from build123d import *

# Parameters (mm, degrees)
F0_R      = 3
F0_R_2    = 15
F1_DEPTH  = 12
F2_R      = 6
F3_DEPTH  = 6
F4_R      = 2
F5_DEPTH  = 12.001
F6_R      = 35
F7_DEPTH  = 4
F8_R      = 35
F9_DEPTH  = 4
F10_R     = 2
F11_DEPTH = 25


with BuildPart() as f1:
    # F0 (on Top) → F1 (new body)
    with BuildSketch(Plane.XY):
        with BuildLine():
            Line((7, 55.425626), (7, 100))
            ThreePointArc((7, 100), (0, 107), (-7, 100))
            Line((-7, 100), (-7, 55.425626))
            ThreePointArc((-7, 55.425626), (-19.5, 33.774991), (-44.5, 33.774991))
            Line((-44.5, 33.774991), (-83.10254, 56.062178))
            ThreePointArc((-83.10254, 56.062178), (-92.664718, 53.5), (-90.10254, 43.937822))
            Line((-90.10254, 43.937822), (-51.5, 21.650635))
            ThreePointArc((-51.5, 21.650635), (-39, 0), (-51.5, -21.650635))
            Line((-51.5, -21.650635), (-90.10254, -43.937822))
            ThreePointArc((-90.10254, -43.937822), (-92.664718, -53.5), (-83.10254, -56.062178))
            Line((-83.10254, -56.062178), (-44.5, -33.774991))
            ThreePointArc((-44.5, -33.774991), (-19.5, -33.774991), (-7, -55.425626))
            Line((-7, -55.425626), (-7, -100))
            ThreePointArc((-7, -100), (0, -107), (7, -100))
            Line((7, -100), (7, -55.425626))
            ThreePointArc((7, -55.425626), (19.5, -33.774991), (44.5, -33.774991))
            Line((44.5, -33.774991), (83.10254, -56.062178))
            ThreePointArc((83.10254, -56.062178), (92.664718, -53.5), (90.10254, -43.937822))
            Line((90.10254, -43.937822), (51.5, -21.650635))
            ThreePointArc((51.5, -21.650635), (39, 0), (51.5, 21.650635))
            Line((51.5, 21.650635), (90.10254, 43.937822))
            ThreePointArc((90.10254, 43.937822), (92.664718, 53.5), (83.10254, 56.062178))
            Line((83.10254, 56.062178), (44.5, 33.774991))
            ThreePointArc((44.5, 33.774991), (19.5, 33.774991), (7, 55.425626))
        make_face()
        with Locations((-86.60254, -50)):
            Circle(F0_R, mode=Mode.SUBTRACT)
        with Locations((-38.971143, -22.5)):
            Circle(F0_R, mode=Mode.SUBTRACT)
        with Locations((0, -100)):
            Circle(F0_R, mode=Mode.SUBTRACT)
        with Locations((0, -45)):
            Circle(F0_R, mode=Mode.SUBTRACT)
        Circle(F0_R_2, mode=Mode.SUBTRACT)
        with Locations((38.971143, -22.5)):
            Circle(F0_R, mode=Mode.SUBTRACT)
        with Locations((86.60254, -50)):
            Circle(F0_R, mode=Mode.SUBTRACT)
        with Locations((-86.60254, 50)):
            Circle(F0_R, mode=Mode.SUBTRACT)
        with Locations((-38.971143, 22.5)):
            Circle(F0_R, mode=Mode.SUBTRACT)
        with Locations((38.971143, 22.5)):
            Circle(F0_R, mode=Mode.SUBTRACT)
        with Locations((0, 45)):
            Circle(F0_R, mode=Mode.SUBTRACT)
        with Locations((86.60254, 50)):
            Circle(F0_R, mode=Mode.SUBTRACT)
        with Locations((0, 100)):
            Circle(F0_R, mode=Mode.SUBTRACT)
    extrude(amount=F1_DEPTH)

    # F2 (on face) → F3 (cut)
    with BuildSketch(Plane.XY.offset(12)):
        with Locations((-86.60254, 50)):
            Circle(F2_R)
        with Locations((0, 100)):
            Circle(F2_R)
        with Locations((86.60254, 50)):
            Circle(F2_R)
        with Locations((86.60254, -50)):
            Circle(F2_R)
        with Locations((0, -100)):
            Circle(F2_R)
        with Locations((-86.60254, -50)):
            Circle(F2_R)
        with Locations((-38.971143, 22.5)):
            Circle(F2_R)
        with Locations((0, 45)):
            Circle(F2_R)
        with Locations((38.971143, 22.5)):
            Circle(F2_R)
        with Locations((38.971143, -22.5)):
            Circle(F2_R)
        with Locations((0, -45)):
            Circle(F2_R)
        with Locations((-38.971143, -22.5)):
            Circle(F2_R)
    extrude(amount=-F3_DEPTH, mode=Mode.SUBTRACT)

    # F4 (on face) → F5 (cut, through all)
    with BuildSketch(Plane.XY.offset(12)):
        with Locations((0, 20)):
            Circle(F4_R)
        with Locations((-20, 0)):
            Circle(F4_R)
        with Locations((0, -20)):
            Circle(F4_R)
        with Locations((20, 0)):
            Circle(F4_R)
    extrude(amount=-F5_DEPTH, mode=Mode.SUBTRACT)

    # F6 (on face) → F7 (cut)
    with BuildSketch(Plane.XY.offset(12)):
        Circle(F6_R)
        with BuildLine():
            ThreePointArc((0, 93), (-3.535534, 91.535534), (-5, 88))
            Line((-5, 88), (-5, 57))
            ThreePointArc((-5, 57), (-3.535534, 53.464466), (0, 52))
            ThreePointArc((0, 52), (3.535534, 53.464466), (5, 57))
            Line((5, 57), (5, 88))
            ThreePointArc((5, 88), (3.535534, 91.535534), (0, 93))
        make_face()
        with BuildLine():
            Line((-46.863448, 32.830127), (-73.710236, 48.330127))
            ThreePointArc((-73.710236, 48.330127), (-77.504331, 48.829629), (-80.540363, 46.5))
            ThreePointArc((-80.540363, 46.5), (-81.039865, 42.705905), (-78.710236, 39.669873))
            Line((-78.710236, 39.669873), (-51.863448, 24.169873))
            ThreePointArc((-51.863448, 24.169873), (-48.069353, 23.670371), (-45.033321, 26))
            ThreePointArc((-45.033321, 26), (-44.533819, 29.794095), (-46.863448, 32.830127))
        make_face()
        with BuildLine():
            Line((-51.863448, -24.169873), (-78.710236, -39.669873))
            ThreePointArc((-78.710236, -39.669873), (-81.039865, -42.705905), (-80.540363, -46.5))
            ThreePointArc((-80.540363, -46.5), (-77.504331, -48.829629), (-73.710236, -48.330127))
            Line((-73.710236, -48.330127), (-46.863448, -32.830127))
            ThreePointArc((-46.863448, -32.830127), (-44.533819, -29.794095), (-45.033321, -26))
            ThreePointArc((-45.033321, -26), (-48.069353, -23.670371), (-51.863448, -24.169873))
        make_face()
        with BuildLine():
            Line((-5, -57), (-5, -88))
            ThreePointArc((-5, -88), (-3.535534, -91.535534), (0, -93))
            ThreePointArc((0, -93), (3.535534, -91.535534), (5, -88))
            Line((5, -88), (5, -57))
            ThreePointArc((5, -57), (3.535534, -53.464466), (0, -52))
            ThreePointArc((0, -52), (-3.535534, -53.464466), (-5, -57))
        make_face()
        with BuildLine():
            Line((46.863448, -32.830127), (73.710236, -48.330127))
            ThreePointArc((73.710236, -48.330127), (77.504331, -48.829629), (80.540363, -46.5))
            ThreePointArc((80.540363, -46.5), (81.039865, -42.705905), (78.710236, -39.669873))
            Line((78.710236, -39.669873), (51.863448, -24.169873))
            ThreePointArc((51.863448, -24.169873), (48.069353, -23.670371), (45.033321, -26))
            ThreePointArc((45.033321, -26), (44.533819, -29.794095), (46.863448, -32.830127))
        make_face()
        with BuildLine():
            Line((51.863448, 24.169873), (78.710236, 39.669873))
            ThreePointArc((78.710236, 39.669873), (81.039865, 42.705905), (80.540363, 46.5))
            ThreePointArc((80.540363, 46.5), (77.504331, 48.829629), (73.710236, 48.330127))
            Line((73.710236, 48.330127), (46.863448, 32.830127))
            ThreePointArc((46.863448, 32.830127), (44.533819, 29.794095), (45.033321, 26))
            ThreePointArc((45.033321, 26), (48.069353, 23.670371), (51.863448, 24.169873))
        make_face()
    extrude(amount=-F7_DEPTH, mode=Mode.SUBTRACT)

    # F8 (on face) → F9 (cut)
    with BuildSketch(Plane(origin=(0, 0, 0), x_dir=(1, 0, 0), z_dir=(0, 0, -1))):
        Circle(F8_R)
        with BuildLine():
            ThreePointArc((-73.710236, 48.330127), (-80.540363, 46.5), (-78.710236, 39.669873))
            Line((-78.710236, 39.669873), (-51.863448, 24.169873))
            ThreePointArc((-51.863448, 24.169873), (-45.033321, 26), (-46.863448, 32.830127))
            Line((-46.863448, 32.830127), (-73.710236, 48.330127))
        make_face()
        with BuildLine():
            ThreePointArc((-78.710236, -39.669873), (-80.540363, -46.5), (-73.710236, -48.330127))
            Line((-73.710236, -48.330127), (-46.863448, -32.830127))
            ThreePointArc((-46.863448, -32.830127), (-45.033321, -26), (-51.863448, -24.169873))
            Line((-51.863448, -24.169873), (-78.710236, -39.669873))
        make_face()
        with BuildLine():
            ThreePointArc((5, -57), (0, -52), (-5, -57))
            Line((-5, -57), (-5, -88))
            ThreePointArc((-5, -88), (0, -93), (5, -88))
            Line((5, -88), (5, -57))
        make_face()
        with BuildLine():
            ThreePointArc((73.710236, -48.330127), (80.540363, -46.5), (78.710236, -39.669873))
            Line((78.710236, -39.669873), (51.863448, -24.169873))
            ThreePointArc((51.863448, -24.169873), (45.033321, -26), (46.863448, -32.830127))
            Line((46.863448, -32.830127), (73.710236, -48.330127))
        make_face()
        with BuildLine():
            ThreePointArc((78.710236, 39.669873), (80.540363, 46.5), (73.710236, 48.330127))
            Line((73.710236, 48.330127), (46.863448, 32.830127))
            ThreePointArc((46.863448, 32.830127), (45.033321, 26), (51.863448, 24.169873))
            Line((51.863448, 24.169873), (78.710236, 39.669873))
        make_face()
        with BuildLine():
            ThreePointArc((5, 88), (0, 93), (-5, 88))
            Line((-5, 88), (-5, 57))
            ThreePointArc((-5, 57), (0, 52), (5, 57))
            Line((5, 57), (5, 88))
        make_face()
    extrude(amount=-F9_DEPTH, mode=Mode.SUBTRACT)

    # F10 (on face) → F11 (cut)
    with BuildSketch(Plane.XY.offset(8)):
        with Locations((14.142136, 14.142136)):
            Circle(F10_R)
    extrude(amount=-F11_DEPTH, mode=Mode.SUBTRACT)


solid = f1.part
Geometry: final body of the model. Coordinates: model frame, mm. A direction names the side the tool comes from. Round coordinates to 2 decimals unless told otherwise and drop trailing zeros. Order: outer loops, then holes, each group sorted by start corner. A loop starts at its lowest first (then second) coordinate and runs counter-clockwise, first axis right, second up.
Q1. Section B-B, the plane x = 65. Output: boundary loops of the cut face in (y, z), and give its area (3 significant figures).
Result sheet:
outline: (-45.61, 0) - (-43.3, 0) - (-43.3, 4) - (-31.75, 4) - (-31.75, 0) - (-29.44, 0) - (-29.44, 12) - (-31.75, 12) - (-31.75, 8) - (-43.3, 8) - (-43.3, 12) - (-45.61, 12) - close; (29.44, 0) - (31.75, 0) - (31.75, 4) - (43.3, 4) - (43.3, 0) - (45.61, 0) - (45.61, 12) - (43.3, 12) - (43.3, 8) - (31.75, 8) - (31.75, 12) - (29.44, 12) - close
area: 203 mm2
Q2. Material intervals for probe 1 along X at (y, z) = (45, 2.4); probe 2 along X at (y, z) = (58.5, 9.5); probe 3 along Y at (x, z) = (67, 2), sorted ascending.
Result sheet:
probe 1: x = -91.5 to -81.11, -67.94 to -63.94, -9.28 to -3, 3 to 9.28, 63.94 to 67.94, 81.11 to 91.5
probe 2: x = -7 to -5, 5 to 7
probe 3: y = -46.77 to -44.46, -32.91 to -30.6, 30.6 to 32.91, 44.46 to 46.77
Q3. Section C-C, the plane y = -75.5. Output: boundary loops of the cut face in (x, z), and give its area (3 significant figures).
Result sheet:
outline: (-7, 0) - (-5, 0) - (-5, 4) - (5, 4) - (5, 0) - (7, 0) - (7, 12) - (5, 12) - (5, 8) - (-5, 8) - (-5, 12) - (-7, 12) - close
area: 88.0 mm2
Q4. Pin query (flat end, axial travel): pin 1 (8 mm diameter, centred on x = 86.6, y = -50, fed in from +Z); pin 2 (1.2 mm diameter, centred on y = -73.5, z = 10, fed in from +X); pin 3 (6 mm diameter, centred on x = 57.5, z = 3.5, fed in from -Y). Return the tip coordinate at first contact, or that it passes through.
Result sheet:
pin 1: stops at z = 6
pin 2: stops at x = 7
pin 3: stops at y = -43.01
Q5. Access query for faces 4 (the face through (-63, 36, 8)), 5 (the face through (70.531, 32.638, 5.916)), 6 (the face through (80.484, 46.595, 1.972)), 7 (the face through (-71.07, 32.95, 5.92)). Directions: +Z, -Z, +X, -X, +Y, -Y. A direction counts if a zero-diameter tool reaches every point of the face in a straight line with its end or side. Return the directions, or none.
Result sheet:
face 4: +Z
face 5: +Z, -Z, +X
face 6: -Z
face 7: +Z, -Z, -X
Q6. Mould query, pull axis X, two halves, no side actions, for faces 1 (the face through (71.07, -32.95, 5.92)), 2 (the face through (-80.484, -46.595, 1.972)), 3 (the face through (0, 107, 6)). Classes: released by +X, released by -X, zero draft, split by the parting line, or undercut.
Result sheet:
face 1: released by +X
face 2: undercut
face 3: split by the parting line
Q7. Section A-A, the plane y = -8.5. Output: boundary loops of the cut face in (x, z), and give its area (3 significant figures).
Result sheet:
outline: (-40.49, 0) - (-33.95, 0) - (-33.95, 4) - (-12.36, 4) - (-12.36, 8) - (-33.95, 8) - (-33.95, 12) - (-40.49, 12) - close; (12.36, 4) - (33.95, 4) - (33.95, 0) - (40.49, 0) - (40.49, 12) - (33.95, 12) - (33.95, 8) - (12.36, 8) - close
area: 330 mm2
